Print and shaded views of the part. All mm, measured from the part's lowest x, y and z. A direction names the side the tool comes from. Round coordinates to 2 decimals unless told otherwise and drop trailing zeros. Order: outer loops, then holes, each group sorted by start corner. A loop starts at its lowest first (then second) coordinate and runs counter-clockwise, first axis right, second up. Notation, with made-up numbers: M -1.5,0 L 21.5,0 A17 cw 21.5,14 Z; hole C 11.5,36 d7. An arc over 180 degrees is marked long. Use CSV: the item, a comma, the result in double quotes.
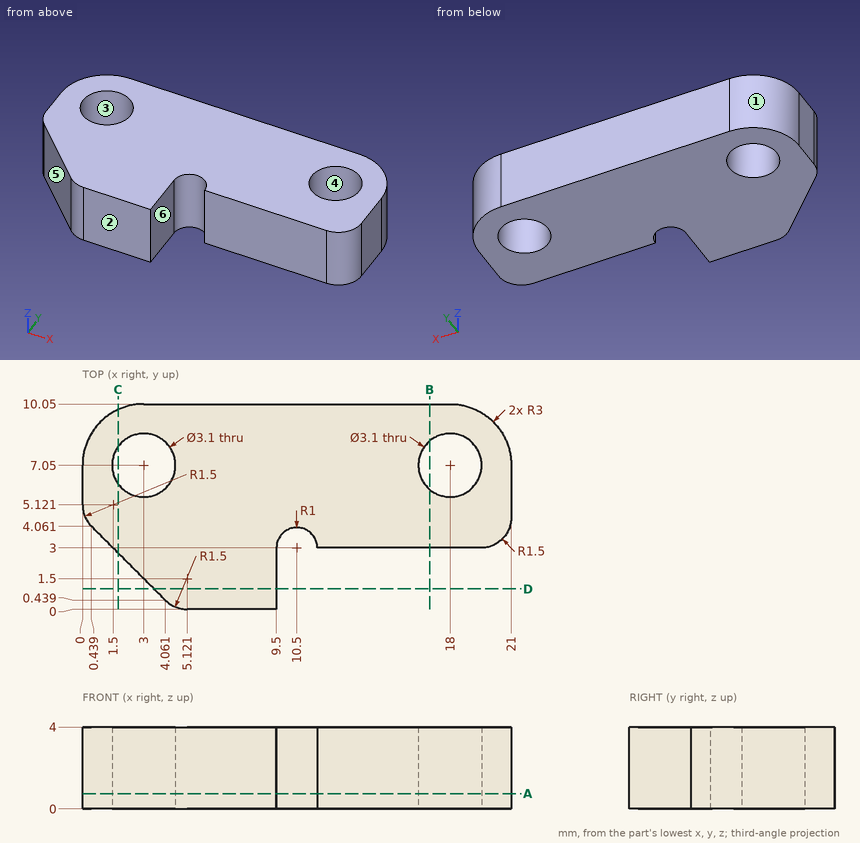
(1) Tool access for the marked faces 5 and 6: list every direction of +Z, -Z, +X, -X, +Y, -Y with a clear straight run to the whole face (end or side of a thin tool).
Answer block:
face 5,"+Z, -Z, -X, -Y"
face 6,"+Z, -Z, +X, -Y"
(2) Two-plate mould, pull along X, no slides. Class the marked faces 1, 2, 3 and 4: released by +X, released by -X, zero draft, split by the parting line, or undercut.
Answer block:
face 1,"released by -X"
face 2,"zero draft"
face 3,"undercut"
face 4,"undercut"
(3) Cut at D-D, the plane y = 1. Give the cut face in (x, z).
Answer block:
outline,"M 3.5,0 L 9.5,0 L 9.5,4 L 3.5,4 Z"
(4) Drop a flat-ended pin along its axis: pin 1 (2 mm diameter, centred on x = 16, z = 2.5, fed in from -Y). Give the stop position or say it passes through.
Answer block:
pin 1,"stops at y = 3"
(5) Cut at C-C, the plane x = 1.75. Give the cut face in (y, z).
Answer block:
outline,"M 2.75,0 L 6.13,0 L 6.13,4 L 2.75,4 Z; M 7.97,0 L 9.78,0 L 9.78,4 L 7.97,4 Z"
(6) Wall check: line 1 (Y direction, x = 18, z = 2.55); line 2 (X direction, y = 8, z = 2.25) (1 decimal); line 3 (Y direction, x = 17.25, z = 1.7). Give the ranges that are in metal, low to high. Write a range as from..to.
Answer block:
line 1,"y = 3..5.5, 8.6..10.05"
line 2,"x = 0.2..1.8, 4.2..16.8, 19.2..20.8"
line 3,"y = 3..5.69, 8.41..10.05"
(7) Cut at B-B, the plane x = 17. Give the cut face in (y, z).
Answer block:
outline,"M 3,0 L 5.87,0 L 5.87,4 L 3,4 Z; M 8.23,0 L 10.05,0 L 10.05,4 L 8.23,4 Z"
(8) Cut at A-A, the plane z = 0.75. Give the cut face in (x, y).
Answer block:
outline,"M 0,5.12 A1.5 ccw 0.44,4.06 L 4.06,0.44 A1.5 ccw 5.12,0 L 9.5,0 L 9.5,3 A1 cw 11.5,3 L 19.5,3 A1.5 ccw 21,4.5 L 21,7.05 A3 ccw 18,10.05 L 3,10.05 A3 ccw 0,7.05 Z; hole C 3,7.05 d3.1; hole C 18,7.05 d3.1"
